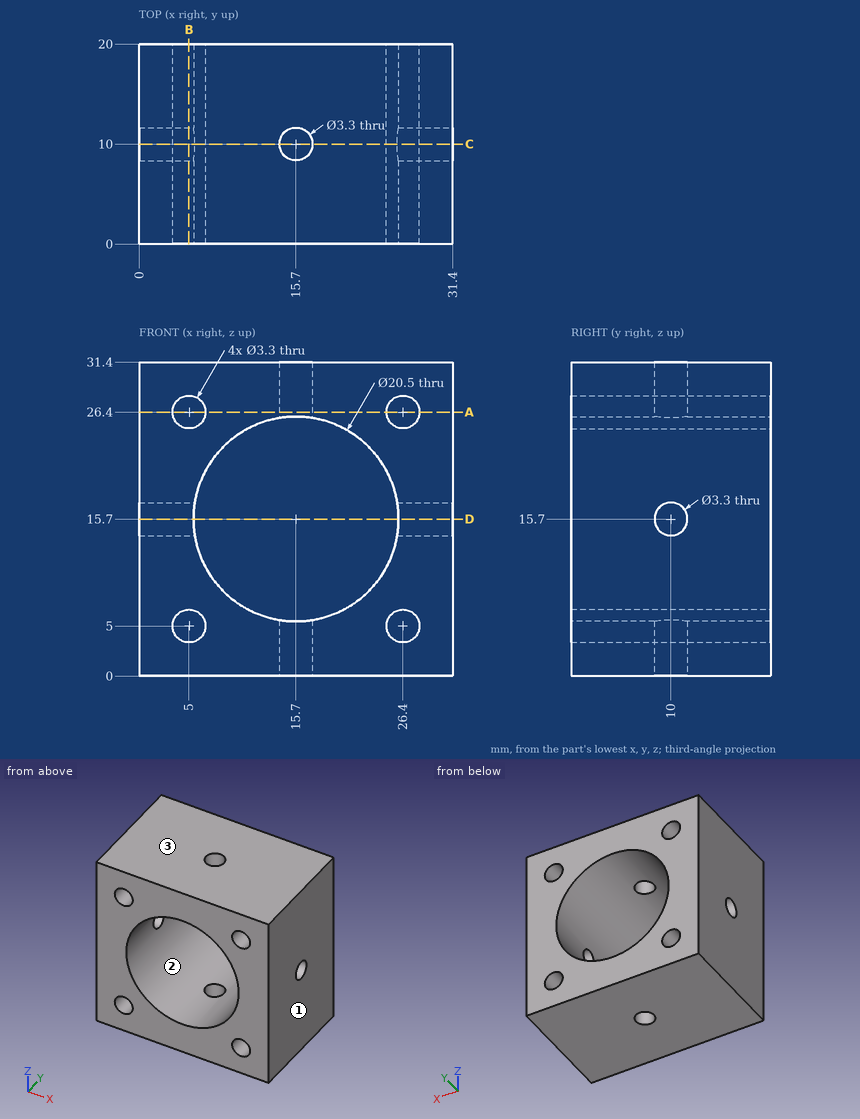
Geometry: see drawing. Coordinates: mm, zero at the bounding-box minimum. Round coordinates to 2 decimals unless told otherwise and drop trailing zeros. Loops run counter-clockwise (first coordinate to the right, second up) from the corner with the lowest first, then second, coordinate; pieces in that order, holes last. Notation, with made-up numbers: M -27.5,27 L 9.5,27 A7 cw 9.5,35 Z; hole C -15,19.25 d8. An arc over 180 degrees is marked long. Use a Markdown table: item, result. Add a question column.
1. Section query B-B on x = 5. Return the cut outline in (y, z).
2. Mould query, pull axis X, two halves, no side actions, for the marked faces 1, 2 and 3. Classes: pulls with the +X half, pulls with the -X half, needs draft (parallel to the pull), parting line crosses it, or undercut.
3. Contact query for flat-ended pins moving along their axis: P1, Ø5.5, axis at x = 26.4, z = 5, coming from the +Y side; P2, Ø4, axis at x = 9.5, z = 18, coming from the -Y side. Output: stop coordinate, or through.
4. Section query D-D on z = 15.7. Return the cut outline in (x, y).
5. Line query: line 1 (X direction, y = 13.5, z = 26.4); line 2 (X direction, y = 12, z = 14); line 3 (X direction, y = 4, z = 25). Output: solid intervals per line, ascending.
6. Section query A-A on z = 26.4. Return the cut outline in (x, y).
7. Section query C-C on y = 10. Return the cut outline in (x, z), then the cut area to 3 significant figures.
Reported:
| question | item | result |
|---|---|---|
| 1 | outline | M 0,0 L 20,0 L 20,3.35 L 0,3.35 Z; M 0,6.65 L 20,6.65 L 20,24.75 L 0,24.75 Z; M 0,28.05 L 20,28.05 L 20,31.4 L 0,31.4 Z; hole C 10,15.7 d3.3 |
| 2 | face 1 | pulls with the +X half |
| 2 | face 2 | undercut |
| 2 | face 3 | needs draft |
| 3 | P1 | stops at y = 20 |
| 3 | P2 | passes through |
| 4 | outline | M 0,0 L 5.45,0 L 5.45,8.35 L 0,8.35 Z; M 0,11.65 L 5.45,11.65 L 5.45,20 L 0,20 Z; M 25.95,0 L 31.4,0 L 31.4,8.35 L 25.95,8.35 Z; M 25.95,11.65 L 31.4,11.65 L 31.4,20 L 25.95,20 Z |
| 5 | line 1 | x = 0 to 3.35, 6.65 to 24.75, 28.05 to 31.4 |
| 5 | line 2 | x = 0 to 5.59, 25.81 to 31.4 |
| 5 | line 3 | x = 0 to 4.13, 5.87 to 11.39, 20.01 to 25.53, 27.27 to 31.4 |
| 6 | outline | M 0,0 L 3.35,0 L 3.35,20 L 0,20 Z; M 6.65,0 L 24.75,0 L 24.75,20 L 6.65,20 Z; M 28.05,0 L 31.4,0 L 31.4,20 L 28.05,20 Z; hole C 15.7,10 d3.3 |
| 7 | outline | M 0,0 L 14.05,0 L 14.05,5.58 A10.25 cw 5.58,14.05 L 0,14.05 Z; M 0,17.35 L 5.58,17.35 A10.25 cw 14.05,25.82 L 14.05,31.4 L 0,31.4 Z; M 17.35,0 L 31.4,0 L 31.4,14.05 L 25.82,14.05 A10.25 cw 17.35,5.58 Z; M 17.35,25.82 A10.25 cw 25.82,17.35 L 31.4,17.35 L 31.4,31.4 L 17.35,31.4 Z; hole C 5,5 d3.3; hole C 5,26.4 d3.3; hole C 26.4,5 d3.3; hole C 26.4,26.4 d3.3 |
| 7 | area | 549 mm² |
